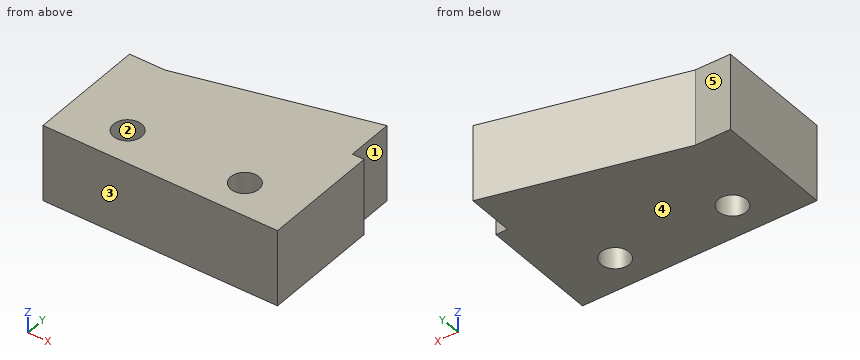
```python
from build123d import *

# Parameters (mm, degrees)
SKETCH1_W            = 20
SKETCH1_H            = 10
BOSS_EXTRUDE1_DEPTH  = 6.5
M2_CLEARANCE_HOLE1_D = 2.4


with BuildPart() as part:
    # Sketch1 → Boss-Extrude1 (new body)
    with BuildSketch(Plane.XY):
        Polygon((19, 14), (3, 10), (19, 10), align=None)
        with Locations((10, 5)):
            Rectangle(SKETCH1_W, SKETCH1_H)
    extrude(amount=BOSS_EXTRUDE1_DEPTH)

    # M2 Clearance Hole1 (through all)
    with Locations(Plane.XY.offset(6.5)):
        with Locations((5, 3), (15, 3)):
            Hole(M2_CLEARANCE_HOLE1_D / 2)


solid = part.part
```
Source: CAD feature listing. Evaluate the final solid. Frame: model axes, mm. Face numbers are marked on the shaded views. A direction names the side the tool comes from. Give positions to 0.01 mm unless a question says otherwise; leave off trailing zeros. Loops run counter-clockwise (first coordinate to the right, second up) from the corner with the lowest first, then second, coordinate; pieces in that order, holes last. Notation, with made-up numbers: (22, 85) -> (33, 85) arc R14 cw to (33, 110) -> close; hole circle Ø7 at (68.5, 65). An arc over 180 degrees is marked (long way). Use a Markdown table: item, result. Add a question column.
(1) Section query B-B (y = 3). Output: boundary loops of the cut face in (x, z).
(2) Ray query, line 1 (Y direction, x = 15, z = 3); line 2 (Y direction, x = 4.5, z = 1) (3 decimals); line 3 (Y direction, x = 1.75, z = 6.25). Return the intervals inside material, ascending.
(3) First-contact query: pin 1 Ø1.2 at (y, z) = (12.5, 4) entering from +X; pin 2 Ø2 at (x, z) = (16, 5.5) entering from -Y; pin 3 Ø2 at (x, z) = (7.5, 5) entering from +Y (3 decimals); pin 4 Ø2 at (x, y) = (15, 3) entering from -Z. Flat tips, straight axial feed; report the tip coordinate or a pass-through.
(4) Access query for the marked faces 4 and 5. Directions: +Z, -Z, +X, -X, +Y, -Y. A direction counts if a zero-diameter tool reaches every point of the face in a straight line with its end or side. Return the directions, or none.
(5) Pull-direction query (Y, two-part tool) for the marked faces 1, 2 and 3; classes: +Y half, -Y half, draft (parallel to the pull), parting line (faces both ways), or undercut.
(6) Section query A-A (x = 5). Output: boundary loops of the cut face in (y, z), then the cut area to 4 significant figures.
(7) Section query D-D (x = 15). Output: boundary loops of the cut face in (y, z).
(8) Section query C-C (z = 3.5). Output: boundary loops of the cut face in (x, y).
Checked values:
| question | item | result |
|---|---|---|
| 1 | outline | (0, 0) -> (3.8, 0) -> (3.8, 6.5) -> (0, 6.5) -> close; (6.2, 0) -> (13.8, 0) -> (13.8, 6.5) -> (6.2, 6.5) -> close; (16.2, 0) -> (20, 0) -> (20, 6.5) -> (16.2, 6.5) -> close |
| 2 | line 1 | 0 to 1.8, 4.2 to 13 |
| 2 | line 2 | 0 to 1.909, 4.091 to 10.375 |
| 2 | line 3 | 0 to 10 |
| 3 | pin 1 | x = 19 |
| 3 | pin 2 | y = 0 |
| 3 | pin 3 | y = 11.375 |
| 3 | pin 4 | through |
| 4 | face 4 | -Z, +X, -X, +Y, -Y |
| 4 | face 5 | +Z, -Z, -X, +Y |
| 5 | face 1 | draft |
| 5 | face 2 | undercut |
| 5 | face 3 | -Y half |
| 6 | outline | (0, 0) -> (1.8, 0) -> (1.8, 6.5) -> (0, 6.5) -> close; (4.2, 0) -> (10.5, 0) -> (10.5, 6.5) -> (4.2, 6.5) -> close |
| 6 | area | 52.65 mm^2 |
| 7 | outline | (0, 0) -> (1.8, 0) -> (1.8, 6.5) -> (0, 6.5) -> close; (4.2, 0) -> (13, 0) -> (13, 6.5) -> (4.2, 6.5) -> close |
| 8 | outline | (0, 0) -> (20, 0) -> (20, 10) -> (19, 10) -> (19, 14) -> (3, 10) -> (0, 10) -> close; hole circle Ø2.4 at (5, 3); hole circle Ø2.4 at (15, 3) |
